Source: CAD feature listing. Evaluate the final solid. Frame: model axes, mm. Give positions to 0.01 mm unless a question says otherwise; leave off trailing zeros.
```python
from build123d import *

# Parameters (mm, degrees)
SKETCH1_W                                       = 600
SKETCH1_H                                       = 180
BOSS_EXTRUDE1_DEPTH                             = 6
CSK_FOR_M4_FLAT_HEAD_MACHINE_SCREW1_D           = 4.3
CSK_FOR_M4_FLAT_HEAD_MACHINE_SCREW1_CSINK_D     = 9.4
CSK_FOR_M4_FLAT_HEAD_MACHINE_SCREW1_CSINK_ANGLE = 90
F_4_0MM_DOWEL_HOLE1_D                           = 4
F_3_0MM_DOWEL_HOLE1_D                           = 3
SKETCH8_R                                       = 5
CUT_EXTRUDE1_DEPTH                              = 10


with BuildPart() as part:
    # Sketch1 → Boss-Extrude1 (new body)
    with BuildSketch(Plane.XY):
        with Locations((300, 90)):
            Rectangle(SKETCH1_W, SKETCH1_H)
    extrude(amount=BOSS_EXTRUDE1_DEPTH)

    # CSK for M4 Flat Head Machine Screw1 (through all)
    with Locations(Plane.XY.offset(6)):
        with Locations((546.25, 20), (590, 63.75), (426.25, 20), (306.25, 20), (186.25, 20), (66.25, 20), (10, 63.75), (590, 143.75), (10, 143.75)):
            CounterSinkHole(CSK_FOR_M4_FLAT_HEAD_MACHINE_SCREW1_D / 2, CSK_FOR_M4_FLAT_HEAD_MACHINE_SCREW1_CSINK_D / 2, counter_sink_angle=CSK_FOR_M4_FLAT_HEAD_MACHINE_SCREW1_CSINK_ANGLE)

    # Ø4.0mm Dowel Hole1 (through all)
    with Locations(Plane.XY.offset(6)):
        with Locations((500, 60), (485, 60), (470, 60), (485, 114), (470, 114), (500, 114), (130, 114), (115, 114), (100, 114), (130, 60), (115, 60), (100, 60)):
            Hole(F_4_0MM_DOWEL_HOLE1_D / 2)

    # Ø3.0mm Dowel Hole1 (through all)
    with Locations(Plane.XY.offset(6)):
        with Locations((532.43, 148.2), (532.43, 168.2), (162.43, 148.2), (162.43, 168.2)):
            Hole(F_3_0MM_DOWEL_HOLE1_D / 2)

    # Sketch8 → Cut-Extrude1 (cut)
    with BuildSketch(Plane.XY.offset(6)):
        with Locations((500, 140)):
            Circle(SKETCH8_R)
        with Locations((130, 140)):
            Circle(SKETCH8_R)
    extrude(amount=-CUT_EXTRUDE1_DEPTH, mode=Mode.SUBTRACT)


solid = part.part
```
1) Draft query along X for faces 1 (the flat face through (296, 91, 6)), 2 (the conical face through (65.028, 21.917, 3.574)). Return one class per face: +X half, -X half, draft (parallel to the pull), parting line (faces both ways), or undercut.
Report:
face 1: draft
face 2: undercut
2) Pin query (flat end, axial travel): pin 1 (7 mm diameter, centred on x = 426.25, y = 20, fed in from +Z); pin 2 (5.5 mm diameter, centred on x = 10, y = 143.75, fed in from +Z). Return the tip coordinate at first contact, or that it passes through.
Report:
pin 1: stops at z = 4.8
pin 2: stops at z = 4.05
3) Material intervals for L1, parallel to X at y = 20, z = 2.6; L2, parallel to Y at x = 10, z = 1; L3, parallel to Y at x = 470, z = 1.55, sorted ascending.
Report:
L1: x = 0 to 64.1, 68.4 to 184.1, 188.4 to 304.1, 308.4 to 424.1, 428.4 to 544.1, 548.4 to 600
L2: y = 0 to 61.6, 65.9 to 141.6, 145.9 to 180
L3: y = 0 to 58, 62 to 112, 116 to 180
